Here's the drawing with two shaded views (mm, measured from the low corner). I have some questions. A direction names the side the tool comes from. Give positions to 0.01 mm unless a question says otherwise; leave off trailing zeros. Loops run counter-clockwise (first coordinate to the right, second up) from the corner with the lowest first, then second, coordinate; pieces in that order, holes last. Notation, with made-up numbers: M 64.25,39.5 L 99.25,39.5 A17 ccw 99.25,68.5 Z; hole C -20.5,48 d11. An arc over 180 degrees is marked long. Write item = value, one per line. Start each with the question number.
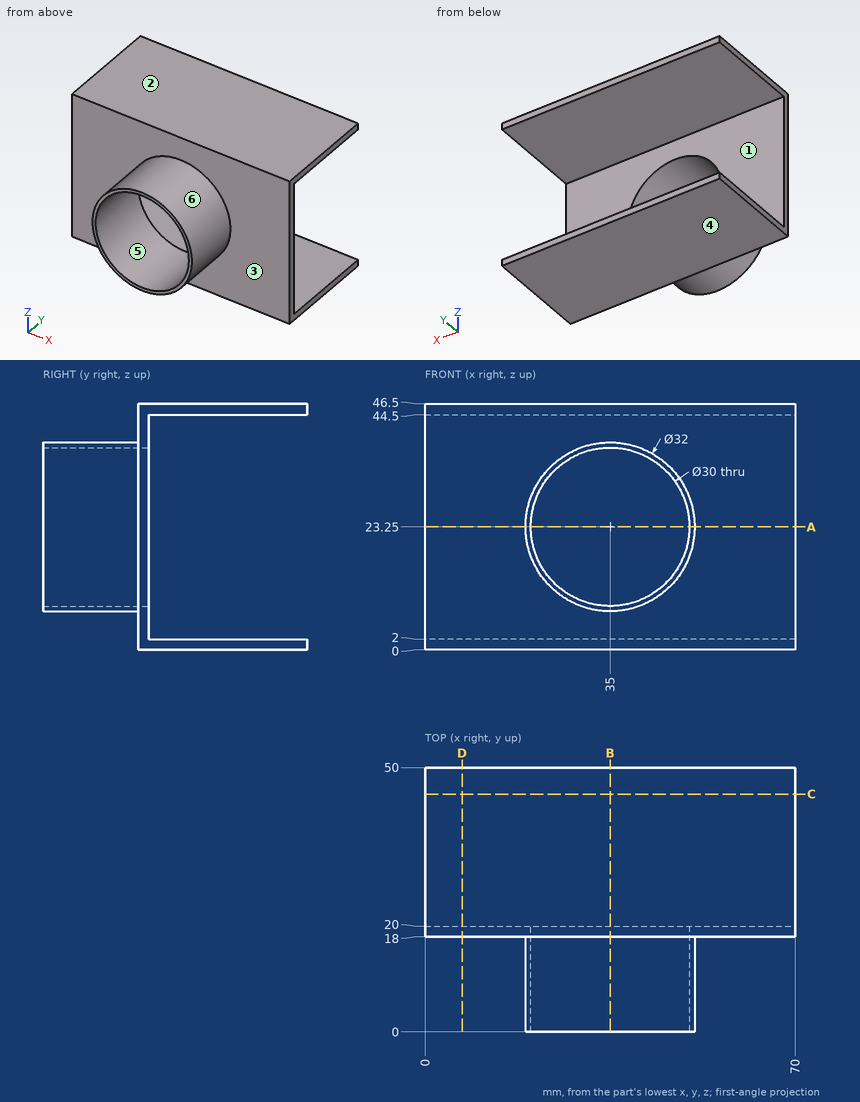
Q1. We'd pull the mould along Z, two halves only. Please class the marked faces 4, 5 and 6: pulls with the +Z half, pulls with the -Z half, needs draft (parallel to the pull), parting line crosses it, or undercut.
Q2. If we section it at C-C, the plane y = 45: List the corners of the cut face in (x, z) for me, then the cut area to 3 significant figures.
Q3. If we section it at A-A, the plane z = 23.25: List the corners of the cut face in (x, y) for me.
Q4. Will these pins go through, and if not, where does the flat tip stop? pin 1 (12 mm diameter, centred on x = 15.5, y = 11, fed in from -Z); pin 2 (8 mm diameter, centred on x = 22, y = 13.5, fed in from -Z); pin 3 (3 mm diameter, centred on x = 49, y = 11.5, fed in from +Z).
Q5. On a 3-axis mill with a long thin cutter (end or side, diameter ignored), from which of +Z, -Z, +X, -X, +Y, -Y can I reach the whole of each face in a straight line? I mean the marked faces 1, 2 and 3. Say none if no direction works.
Q6. If we section it at D-D, the plane x = 7: List the corners of the cut face in (y, z) for me.
Q7. If we section it at B-B, the plane x = 35: List the corners of the cut face in (y, z) for me.
Q8. If I drill on line 1 along Z through (x, y) = (50, 46.5); line 2 along X through (y, z) = (6.5, 23.25); line 3 along Z through (x, y) = (35, 10.75), over which ranges is the centre line in solid material (lowest first)?
Resolved:
q1.face_4 = pulls with the -Z half
q1.face_5 = undercut
q1.face_6 = parting line crosses it
q2.outline = M 0,0 L 70,0 L 70,2 L 0,2 Z; M 0,44.5 L 70,44.5 L 70,46.5 L 0,46.5 Z
q2.area = 280 mm²
q3.outline = M 0,18 L 19,18 L 19,0 L 20,0 L 20,20 L 0,20 Z; M 50,0 L 51,0 L 51,18 L 70,18 L 70,20 L 50,20 Z
q4.pin_1 = 14.66
q4.pin_2 = 10.02
q4.pin_3 = 33.24
q5.face_1 = +X, -X, +Y
q5.face_2 = +Z, +X, -X, +Y, -Y
q5.face_3 = -Y
q6.outline = M 18,0 L 50,0 L 50,2 L 20,2 L 20,44.5 L 50,44.5 L 50,46.5 L 18,46.5 Z
q7.outline = M 0,7.25 L 18,7.25 L 18,0 L 50,0 L 50,2 L 20,2 L 20,8.25 L 0,8.25 Z; M 0,38.25 L 20,38.25 L 20,44.5 L 50,44.5 L 50,46.5 L 18,46.5 L 18,39.25 L 0,39.25 Z
q8.line_1 = 0 to 2, 44.5 to 46.5
q8.line_2 = 19 to 20, 50 to 51
q8.line_3 = 7.25 to 8.25, 38.25 to 39.25
